Source: three-view drawing plus pictorial views. Frame: mm from the lowest corner of the part. A direction names the side the tool comes from. Give positions to 0.01 mm unless a question says otherwise; leave off trailing zeros. Order: outer loops, then holes, each group sorted by start corner. A loop starts at its lowest first (then second) coordinate and runs counter-clockwise, first axis right, second up.
1) First-contact query: P1, Ø15, axis at x = 630, y = 33.5, coming from the -Z side; P2, Ø1.5, axis at y = 24.5, z = 411.5, coming from the -X side; P3, Ø15, axis at y = 23, z = 225.5, coming from the +X side; P4, Ø5, axis at x = 611, z = 509, coming from the -Y side. Flat tips, straight axial feed; report the tip coordinate or a pass-through.
2) Section D-D, the plane x = 432. Return loops of the section in (y, z), plus the area to 3 significant figures.
3) Section A-A, the plane z = 149.5. Return loops of the section in (x, y), plus the area to 3 significant figures.
4) Section B-B, the plane y = 104. Return loops of the section in (x, z), plus the area to 3 significant figures.
5) Access query for the marked faces 1 and 2. Directions: +Z, -Z, +X, -X, +Y, -Y. A direction counts if a zero-diameter tool reaches every point of the face in a straight line with its end or side. Return the directions, or none.
6) Material intervals for line 1 (X direction, y = 112, z = 138); line 2 (X direction, y = 12, z = 158); line 3 (Z direction, x = 272, y = 54), sorted ascending.
7) Section C-C, the plane x = 655.5. Return loops of the section in (y, z).
8) Draft query along X for the marked faces 3, 4 and 5. Return one class per face: released by +X, released by -X, zero draft, split by the parting line, or undercut.
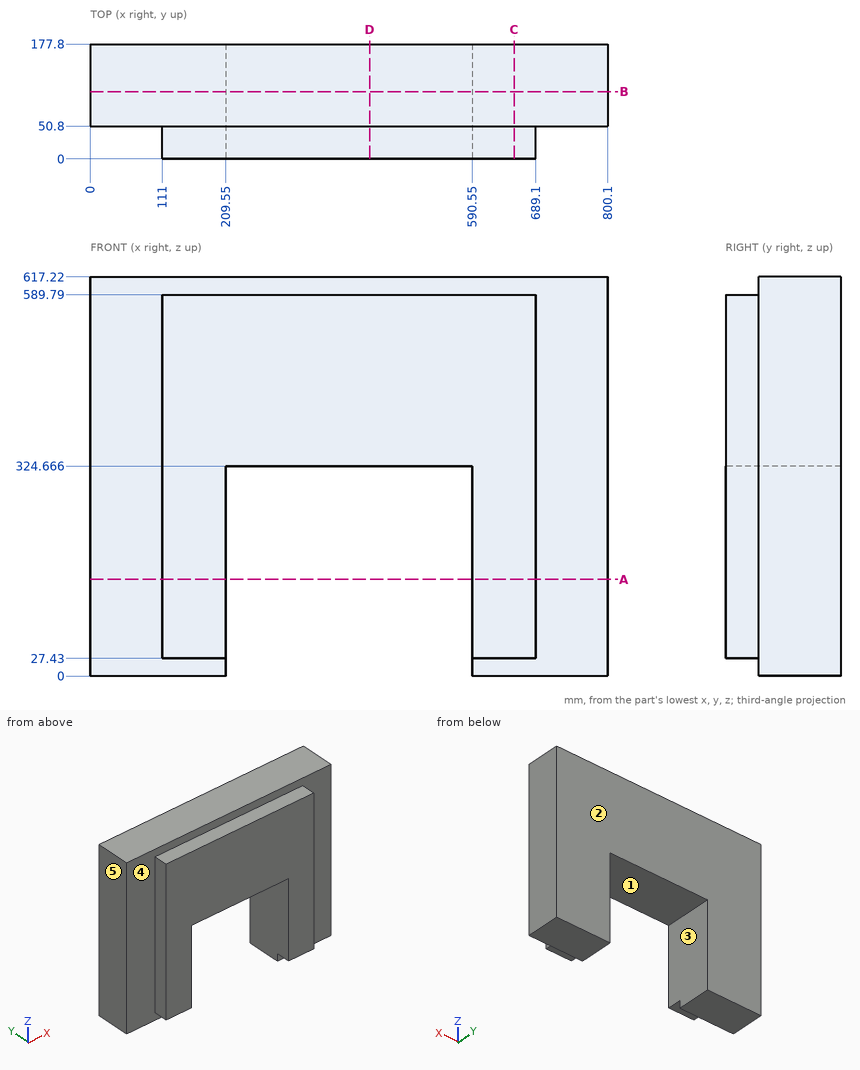
From the geometry:
1. P1: stops at z = 27.43
1. P2: stops at x = 111
1. P3: stops at x = 689.1
1. P4: stops at y = 0
2. outline: (0, 324.67) - (177.8, 324.67) - (177.8, 617.22) - (50.8, 617.22) - (50.8, 589.79) - (0, 589.79) - close
2. area: 50,600 mm2
3. outline: (0, 50.8) - (111, 50.8) - (111, 0) - (209.55, 0) - (209.55, 177.8) - (0, 177.8) - close; (590.55, 0) - (689.1, 0) - (689.1, 50.8) - (800.1, 50.8) - (800.1, 177.8) - (590.55, 177.8) - close
3. area: 63,200 mm2
4. outline: (0, 0) - (209.55, 0) - (209.55, 324.67) - (590.55, 324.67) - (590.55, 0) - (800.1, 0) - (800.1, 617.22) - (0, 617.22) - close
4. area: 370,000 mm2
5. face 1: -Z, +Y, -Y
5. face 2: +Z, -Z, +X, -X, +Y
6. line 1: x = 0 to 209.55, 590.55 to 800.1
6. line 2: x = 111 to 209.55, 590.55 to 689.1
6. line 3: z = 324.67 to 617.22
7. outline: (0, 27.43) - (50.8, 27.43) - (50.8, 0) - (177.8, 0) - (177.8, 617.22) - (50.8, 617.22) - (50.8, 589.79) - (0, 589.79) - close
8. face 3: undercut
8. face 4: zero draft
8. face 5: released by -X
